```python
from build123d import *

# Parameters (mm, degrees)
BOSS_EXTRUDE1_DEPTH = 40.64
SKETCH6_R           = 1.1303
CUT_EXTRUDE1_DEPTH  = 158.779215984
SKETCH7_W           = 195.523307817
SKETCH7_H           = 195.523307817
CUT_EXTRUDE2_DEPTH  = 158.779215984
SKETCH8_R           = 1.1303
CUT_EXTRUDE3_DEPTH  = 158.779215984
SKETCH9_R           = 19.05
CUT_EXTRUDE4_DEPTH  = 158.779215984


with BuildPart() as part:
    # Sweep3: sweep along a path in Sketch2
    with BuildLine(Plane.XY) as sweep3_path:
        Line((-111.378641457, -46.568583299), (-11.322173751, -64.21123815))
        ThreePointArc((-11.322173751, -64.21123815), (53.410187761, -37.398216088), (56.466415172, 32.6009))
        Line((56.466415172, 32.6009), (37.416415172, 65.596467884))
    # 3DSketch1 → Sweep3 (sweep)
    with BuildSketch(Plane(origin=(-117.024291009, -78.586652965, -20.32), x_dir=(0.051794909001673446, 0.2937435257699459, 0.9544799780350292), z_dir=(0.984807753012208, -0.17364817766693055, 0))):
        Polygon((0, 0), (3.788092413, -12.121895721), (42.57815872, 0), (38.790066307, 12.121895721), align=None)
    sweep(path=sweep3_path.line)

    # Sketch5 → Boss-Extrude1 (add)
    with BuildSketch(Plane.XY.offset(20.32)):
        with BuildLine():
            Line((-16.967823303, -96.229307816), (-117.024291009, -78.586652965))
            Line((-117.024291009, -78.586652965), (-117.024291009, -97.7138))
            Line((-117.024291009, -97.7138), (3.02e-07, -97.7138))
            ThreePointArc((3.02e-07, -97.7138), (-8.516318665, -97.341969504), (-16.967823303, -96.229307816))
        make_face()
        with BuildLine():
            ThreePointArc((97.7138, -9e-08), (69.09409067, -69.094090521), (3.02e-07, -97.7138))
            Line((3.02e-07, -97.7138), (97.7138, -97.7138))
            Line((97.7138, -97.7138), (97.7138, -9e-08))
        make_face()
        with BuildLine():
            ThreePointArc((84.6226331, 48.8569), (94.384283017, 25.290192366), (97.7138, -9e-08))
            Line((97.7138, -9e-08), (97.7138, 81.852467884))
            Line((97.7138, 81.852467884), (65.5726331, 81.852467884))
            Line((65.5726331, 81.852467884), (84.6226331, 48.8569))
        make_face()
    extrude(amount=-BOSS_EXTRUDE1_DEPTH)

    # Sketch6 → Cut-Extrude1 (cut, through all)
    with BuildSketch(Plane.XY.offset(20.32)):
        with Locations((91.3638, -91.3638)):
            Circle(SKETCH6_R)
        with Locations((-41.9735, -91.3638)):
            Circle(SKETCH6_R)
    extrude(amount=-CUT_EXTRUDE1_DEPTH, mode=Mode.SUBTRACT)

    # Sketch7 → Cut-Extrude2 (cut, through all)
    with BuildSketch(Plane.XY.offset(20.32)):
        with Locations((44.2373629, 0.047853909)):
            Rectangle(SKETCH7_W, SKETCH7_H)
    extrude(amount=-CUT_EXTRUDE2_DEPTH, mode=Mode.SUBTRACT)

    # Sketch8 → Cut-Extrude3 (cut, through all)
    with BuildSketch(Plane.XY.offset(20.32)):
        with Locations((-59.874291009, -91.3638)):
            Circle(SKETCH8_R)
    extrude(amount=-CUT_EXTRUDE3_DEPTH, mode=Mode.SUBTRACT)

    # Sketch9 → Cut-Extrude4 (cut, through all)
    with BuildSketch(Plane.XY.offset(20.32)):
        with Locations((-117.024291009, -97.7138)):
            Circle(SKETCH9_R)
    extrude(amount=-CUT_EXTRUDE4_DEPTH, mode=Mode.SUBTRACT)


solid = part.part
```
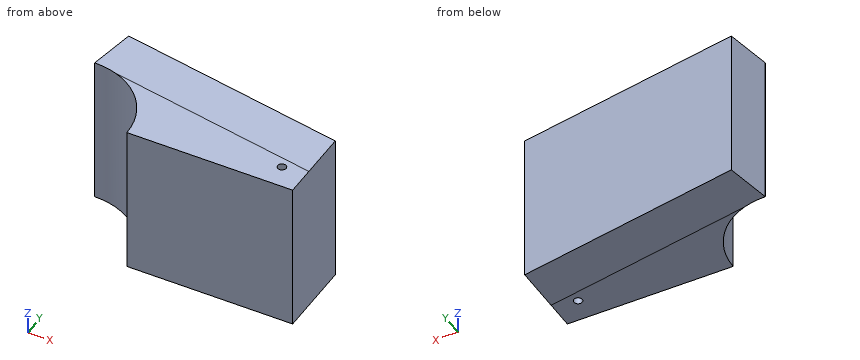
Source: CAD feature listing. Evaluate the final solid. Frame: model axes, mm. Coordinates: 2 decimals unless noted, no trailing zeros. Loops run counter-clockwise (first coordinate to the right, second up) from the corner with the lowest first, then second, coordinate; pieces in that order, holes last. Notation, with made-up numbers: (25, 82.25) - (29, 82.25) arc R16 ccw to (29, 109.25) - close; hole circle Ø10 at (-36.75, -20.75). An arc over 180 degrees is marked (long way). Answer as CSV lines item,"result".
1. Section B-B (x = -74). Return loops of the section in (y, z), then the cut area to 3 significant figures.
Established:
outline,"(-97.71, -20.32) - (-73.28, -20.32) - (-73.28, 20.32) - (-97.71, 20.32) - close"
area,"993 mm2"
2. Contact query for flat-ended pins moving along their axis: pin 1 (1 mm diameter, centred on x = -85, z = 16, fed in from +Y); pin 2 (1.5 mm diameter, centred on y = -78.5, z = -16, fed in from -X); pin 3 (12 mm diameter, centred on y = -88, z = 4, fed in from -X); pin 4 (3 mm diameter, centred on y = -90, z = 12, fed in from -X). Output: stop coordinate, or through.
Established:
pin 1,"stops at y = -71.25"
pin 2,"stops at x = -117.02"
pin 3,"stops at x = -106.25"
pin 4,"stops at x = -100.35"
3. Section A-A (z = 7.5). Return loops of the section in (x, y), then the cut area to 3 significant figures.
Established:
outline,"(-117.02, -78.66) arc R19.05 cw to (-97.97, -97.71) - (-53.52, -97.71) - (-53.52, -76.89) - (-114.82, -66.08) - (-117.02, -78.59) - close; hole circle Ø2.26 at (-59.87, -91.36)"
area,"1,370 mm2"
4. Ray query, line 1 (Y direction, x = -73, z = -17); line 2 (Y direction, x = -66, z = -3.5); line 3 (X direction, y = -82.5, z = 5). Return the intervals inside material, ascending.
Established:
line 1,"y = -97.71 to -73.45"
line 2,"y = -97.71 to -74.69"
line 3,"x = -105.56 to -53.52"
5. Section D-D (y = -71). Return loops of the section in (x, z), then the cut area to 3 significant figures.
Established:
outline,"(-115.69, -20.32) - (-86.91, -20.32) - (-86.91, 20.32) - (-115.69, 20.32) - close"
area,"1,170 mm2"
6. Section C-C (y = -80.5). Return loops of the section in (x, z).
Established:
outline,"(-108.86, -20.32) - (-53.52, -20.32) - (-53.52, 20.32) - (-108.86, 20.32) - close"
